Work out the finished part from the listing and answer in its coordinate system (mm). A direction names the side the tool comes from. Round coordinates to 2 decimals unless told otherwise and drop trailing zeros. Order: outer loops, then holes, each group sorted by start corner. A loop starts at its lowest first (then second) coordinate and runs counter-clockwise, first axis right, second up. Notation, with made-up numbers: (63.5, -31.5) - (121.5, -31.5) arc R22 ccw to (121.5, -10.5) - close; hole circle Ø10 at (38, 86.5). An arc over 180 degrees is marked (long way). Answer in a Markdown table with one row per item.
Autodesk Inventor part; units mm, degrees
ref_plane "YZ Plane" through (0, 0, 0) normal (1, 0, 0) x (0, 1, 0)
ref_plane "XZ Plane" through (0, 0, 0) normal (0, 1, 0) x (-1, 0, 0)
ref_plane "XY Plane" through (0, 0, 0) normal (0, 0, 1) x (1, 0, 0)
sketch "スケッチ1" plane through (0, 0, 0) normal (0, 0, 1) x (1, 0, 0)
  line L0 (-10, -20) -> (10, -20)
  line L1 (10, -20) -> (10, 20)
  line L2 (10, 20) -> (-10, 20)
  line L3 (-10, 20) -> (-10, -20)
  line L4 (-10, -20) -> (10, 20) construction
  line L5 (10, -20) -> (-10, 20) construction
  point P0 (0, 0)
  dimension "d0" = 20
  dimension "d1" = 40
extrude "押し出し1" add sketch "スケッチ1" along normal blind 10
sketch "スケッチ2" plane through (0, 0, 10) normal (0, 0, 1) x (1, 0, 0)
  line L0 (-10, 20) -> (-10, -20)
  line L1 (-10, -20) -> (10, -20)
  line L2 (10, -20) -> (10, 20)
  line L3 (10, 20) -> (-10, 20)
  line L4 (10, 20) -> (-10, 20)
  line L5 (-10, 20) -> (-10, 12.5)
  line L6 (-10, 12.5) -> (10, 12.5)
  line L7 (10, 12.5) -> (10, 20)
  line L8 (10, -20) -> (-10, -20)
  line L9 (-10, -20) -> (-10, -12.5)
  line L10 (-10, -12.5) -> (10, -12.5)
  line L11 (10, -12.5) -> (10, -20)
  line L12 (-10, 20) -> (-2, 20)
  line L13 (-2, 20) -> (-2, -20)
  line L14 (-2, -20) -> (-10, -20)
  line L15 (-10, -20) -> (-10, 20)
  point P0 (0, 0)
  point P1 (10, -12.5)
  point P2 (-2, -12.5)
  point P3 (-2, 12.5)
  point P4 (10, 12.5)
  dimension "d4" = 7.5
  dimension "d5" = 7.5
  dimension "d6" = 8
extrude "押し出し2" add sketch "スケッチ2" along normal blind 40 contours L3 L13 L6 L0 | L6 L13 L10 L0 | L3 L2 L6 L13 | L10 L13 L1 L0 | L10 L2 L1 L13
sketch "スケッチ3" plane through (0, 0, 50) normal (0, 0, 1) x (1, 0, 0)
  line L0 (-10, -20) -> (10, -20)
  line L1 (10, -20) -> (10, -12.5)
  line L2 (10, 12.5) -> (10, 20)
  line L3 (10, 20) -> (-10, 20)
  line L4 (-10, 20) -> (-10, -20)
  line L5 (10, 12.5) -> (-2, 12.5)
  line L6 (-2, 12.5) -> (-2, -12.5)
  line L7 (-2, -12.5) -> (10, -12.5)
  line L8 (10, -12.5) -> (10, 12.5)
  point P0 (0, 0)
extrude "押し出し3" add sketch "スケッチ3" along normal blind 10
sketch "スケッチ4" plane through (0, 0, 60) normal (0, 0, 1) x (1, 0, 0)
  line L0 (10, -20) -> (10, 20)
  point P0 (0, 0)
  point P1 (3, 7.5)
  point P2 (3, -7.5)
  dimension "d11" = 7
  dimension "d12" = 15
  dimension "d13" = 7.5
hole "穴1" at (3, 7.5, 60) at (3, -7.5, 60) direction (0, 0, -1) diameter 3.3 depth 40.25
chamfer "面取り1" distance 10 angle 45 2 edges at (0, 20, 60) (0, -20, 60)
properties part number "Print_Parts_Q" material "PC/ABS プラスチック"
1) The mould has two halves that part along Y. Classify faces 4 (the face through (0, 15, 55)), 5 (the face through (0, 0, 0)), 6 (the face through (4, 0, 50)), 7 (the face through (4, 12.5, 30)): released by +Y, released by -Y, zero draft, split by the parting line, or undercut.
Filled in:
| item | result |
|---|---|
| face 4 | released by +Y |
| face 5 | zero draft |
| face 6 | undercut |
| face 7 | undercut |
2) Find section C-C, the plane z = 23. Give the vertices of the cut face in (x, y), then the cut area to 3 significant figures.
Filled in:
| item | result |
|---|---|
| outline | (-10, -20) - (10, -20) - (10, -12.5) - (-2, -12.5) - (-2, 12.5) - (10, 12.5) - (10, 20) - (-10, 20) - close |
| area | 500 mm^2 |
3) Which of the six approach directions +Z, -Z, +X, -X, +Y, -Y give full straight-line access (tool end or side, diameter ignored) to faces 1 (the face through (2.93, 9.15, 54.93)), 2 (the face through (-2, 0, 30)), 3 (the face through (-10, 0, 30))?
Filled in:
| item | result |
|---|---|
| face 1 | +Z |
| face 2 | +X |
| face 3 | +Z, -Z, -X, +Y, -Y |
4) Find section A-A, the plane y = -7.5. Give the vertices of the cut face in (x, z).
Filled in:
| item | result |
|---|---|
| outline | (-10, 0) - (10, 0) - (10, 10) - (-2, 10) - (-2, 50) - (1.35, 50) - (1.35, 60) - (-10, 60) - close; (4.65, 50) - (10, 50) - (10, 60) - (4.65, 60) - close |
5) Find section B-B, the plane x = 3. Give the vertices of the cut face in (y, z).
Filled in:
| item | result |
|---|---|
| outline | (-20, 0) - (20, 0) - (20, 50) - (10, 60) - (9.15, 60) - (9.15, 50) - (12.5, 50) - (12.5, 10) - (-12.5, 10) - (-12.5, 50) - (-9.15, 50) - (-9.15, 60) - (-10, 60) - (-20, 50) - close; (-5.85, 50) - (5.85, 50) - (5.85, 60) - (-5.85, 60) - close |
6) Find the intervals of material crossed by probe 1 along Y at (x, z) = (7.25, 19); probe 2 along X at (y, z) = (-7.5, 58.25); probe 3 along Z at (x, y) = (0.75, -7), in increasing order. Write a range as from..to.
Filled in:
| item | result |
|---|---|
| probe 1 | y = -20..-12.5, 12.5..20 |
| probe 2 | x = -10..1.35, 4.65..10 |
| probe 3 | z = 0..10, 50..60 |
7) Find section D-D, the plane x = 0.25. Give the vertices of the cut face in (y, z), then the cut area to 3 significant figures.
Filled in:
| item | result |
|---|---|
| outline | (-20, 0) - (20, 0) - (20, 50) - (10, 60) - (-10, 60) - (-20, 50) - close; hole (-12.5, 10) - (12.5, 10) - (12.5, 50) - (-12.5, 50) - close |
| area | 1,300 mm^2 |
